Work out the finished part from the listing and answer in its coordinate system (mm). A direction names the side the tool comes from. Give positions to 0.01 mm unless a question says otherwise; leave off trailing zeros. Order: outer loops, then holes, each group sorted by start corner. A loop starts at its lowest first (then second) coordinate and runs counter-clockwise, first axis right, second up. Notation, with made-up numbers: M -39,65.5 L 16,65.5 A19 cw 16,101.5 Z; hole C -30,39 d2. An arc over 180 degrees is marked long. One line per item, written item: value.
from build123d import *
from OCP.BRepFilletAPI import BRepFilletAPI_MakeChamfer

# Parameters (mm, degrees)
BOSS_EXTRUDE1_DEPTH       = 4
BOSS_EXTRUDE2_DEPTH       = 8
M6X1_0_TAPPED_HOLE1_D     = 5
M6X1_0_TAPPED_HOLE1_DEPTH = 11
M6X1_0_TAPPED_HOLE1_TIP   = 1.502151548
CHAMFER1_SIZE             = 1
CHAMFER1_SIZE2            = 3.732050808
FILLET1_R                 = 1
FILLET2_R                 = 0.5


with BuildPart() as part:
    # Sketch1 → Boss-Extrude1 (new, symmetric)
    with BuildSketch(Plane(origin=(0, 0, 0), x_dir=(1, 0, 0), z_dir=(0, 1, 0))):
        with BuildLine():
            Line((-20, 0), (0, 0))
            Line((0, 0), (20, 0))
            Line((20, 0), (20, -2.8))
            Line((20, -2.8), (24, -2.8))
            Line((24, -2.8), (24, -14.220649169))
            ThreePointArc((24, -14.220649169), (0, -13.5), (-24, -14.220649169))
            Line((-24, -14.220649169), (-24, -2.8))
            Line((-24, -2.8), (-20, -2.8))
            Line((-20, -2.8), (-20, 0))
        make_face()
    extrude(amount=BOSS_EXTRUDE1_DEPTH, both=True)

    # Sketch5 → Boss-Extrude2 (add)
    with BuildSketch(Plane(origin=(0, 4, 0), x_dir=(1, 0, 0), z_dir=(0, 1, 0))):
        Polygon((-20, 16), (-15.6, 16), (-15.6, 0), (-20, 0), (-20, -2.8), (-24, -2.8), align=None)
        Polygon((20, -2.8), (20, 0), (15.6, 0), (15.6, 16), (20, 16), (24, -2.8), align=None)
    extrude(amount=-BOSS_EXTRUDE2_DEPTH)

    # M6x1.0 Tapped Hole1
    with Locations(Plane(origin=(0, 0, 0), x_dir=(-1, 0, 0), z_dir=(0, 0, -1))):
        with Locations((0, 0)):
            Hole(M6X1_0_TAPPED_HOLE1_D / 2, depth=M6X1_0_TAPPED_HOLE1_DEPTH)
            with Locations((0, 0, -(M6X1_0_TAPPED_HOLE1_DEPTH + M6X1_0_TAPPED_HOLE1_TIP / 2))):  # 118° drill point
                Cone(0, M6X1_0_TAPPED_HOLE1_D / 2, M6X1_0_TAPPED_HOLE1_TIP, mode=Mode.SUBTRACT)

    # Chamfer1: one chamfer whose edges measure the first distance from different faces: ONE call of the kernel's chamfer builder (chamfer() names one face for all edges)
    chamfer1_edges_1 = [part.edges().sort_by_distance(p)[0] for p in [
        (-15.6, 0, -16),
    ]]
    chamfer1_side_1 = [part.faces().sort_by_distance(p)[0] for p in [
        (-17.8, 0, -16),
    ]]
    chamfer1_edges_2 = [part.edges().sort_by_distance(p)[0] for p in [
        (15.6, 0, -16),
    ]]
    chamfer1_side_2 = [part.faces().sort_by_distance(p)[0] for p in [
        (17.8, 0, -16),
    ]]
    chamfer1 = BRepFilletAPI_MakeChamfer(part.part.solid().wrapped)
    for e in chamfer1_edges_1:
        chamfer1.Add(CHAMFER1_SIZE, CHAMFER1_SIZE2, e.wrapped, chamfer1_side_1[0].wrapped)  # the first distance lies on this face
    for e in chamfer1_edges_2:
        chamfer1.Add(CHAMFER1_SIZE, CHAMFER1_SIZE2, e.wrapped, chamfer1_side_2[0].wrapped)  # the first distance lies on this face
    add(Compound.cast(chamfer1.Shape()), mode=Mode.REPLACE)

    # Fillet1
    fillet1_edges = [part.edges().sort_by_distance(p)[0] for p in [
        (24, 0, 2.8),
        (-24, 0, 2.8),
        (-20, 0, -16),
        (20, 0, -16),
        (16.6, 0, -16),
        (15.6, 0, -12.267949192),
        (-15.6, 0, -12.267949192),
        (-16.6, 0, -16),
    ]]
    fillet(fillet1_edges, radius=FILLET1_R)

    # Fillet2
    fillet2_edges = [part.edges().sort_by_distance(p)[0] for p in [
        (24, 0, 14.220649169),
        (-24, 0, 14.220649169),
        (-15.6, 0, 0),
        (15.6, 0, 0),
    ]]
    fillet(fillet2_edges, radius=FILLET2_R)


solid = part.part
(1) Section D-D, the plane x = 14 is taken. Give the vertices of the cut face in (y, z), then the cut area to 3 significant figures.
Findings:
outline: M -4,0 L 4,0 L 4,13.75 L -4,13.75 Z
area: 110 mm^2
(2) Section B-B, the plane z = 7 is taken. Give the vertices of the cut face in (x, y), then the cut area to 3 significant figures.
Findings:
outline: M -24,-4 L 24,-4 L 24,4 L -24,4 Z; hole C 0,0 d5
area: 364 mm^2
(3) Section A-A, the plane y = 3.5 is taken. Give the vertices of the cut face in (x, z), then the cut area to 3 significant figures.
Findings:
outline: M -24,2.91 A1 ccw -23.98,2.7 L -20.17,-15.21 A1 ccw -19.19,-16 L -17.37,-16 A1 ccw -16.4,-15.26 L -15.63,-12.4 A1 ccw -15.6,-12.14 L -15.6,-0.5 A0.5 cw -15.1,0 L 15.1,0 A0.5 cw 15.6,-0.5 L 15.6,-12.14 A1 ccw 15.63,-12.4 L 16.4,-15.26 A1 ccw 17.37,-16 L 19.19,-16 A1 ccw 20.17,-15.21 L 23.98,2.7 A1 ccw 24,2.91 L 24,13.69 A0.5 ccw 23.47,14.19 A400 cw -23.47,14.19 A0.5 ccw -24,13.69 Z
area: 849 mm^2
(4) Find the intervals of material crossed by probe 1 along Y at (x, z) = (0, 6); probe 2 along X at (y, z) = (0, 6); probe 3 along X at (y, z) = (1.5, 2.5), in increasing order. Write a range as from..to.
Findings:
probe 1: y = -4..-2.5, 2.5..4
probe 2: x = -24..-2.5, 2.5..24
probe 3: x = -23.94..-2, 2..23.94
(5) Which of the six approach directions +Z, -Z, +X, -X, +Y, -Y give full straight-line access (tool end or side, diameter ignored) to faces 1 (the flat face through (0, 4, 2)), 2 (the flat face through (-15.6, 0, -6)), 3 (the cylindrical face through (-0.54, -2.44, 5.58))?
Findings:
face 1: +Z, -Z, +X, -X, +Y
face 2: -Z, +Y, -Y
face 3: -Z
(6) Determine the mould class of faces 4 (the flat face through (22.047, 0.056, -6.381)), 5 (the cylindrical face through (16.751, -0.056, -15.788)), 6 (the flat face through (18, 0, -16)) for opening direction X: pulls with the +X half, pulls with the -X half, needs draft (parallel to the pull), parting line crosses it, or undercut.
Findings:
face 4: pulls with the +X half
face 5: undercut
face 6: needs draft
(7) Section C-C, the plane x = -9 is taken. Give the vertices of the cut face in (y, z).
Findings:
outline: M -4,0 L 4,0 L 4,13.6 L -4,13.6 Z
(8) Given P1, Ø2.5, axis at y = -0.5, z = -8.5, coming from the -X side; P2, Ø1, axis at y = 0.5, z = -0.5, coming from the +X side; P3, Ø1.5, axis at y = 1, z = -6.5, coming from the +X side, each flat-ended and moving along its own axis, determine where each tip first touches the part or whether it passes through.
Findings:
P1: stops at x = -21.86
P2: stops at x = 23.4
P3: stops at x = 22.18
